Check sheet for the modelled part. Datum: model origin and axes. Units: mm. Coordinates: 2 decimals unless noted, no trailing zeros. Loops run counter-clockwise (first coordinate to the right, second up) from the corner with the lowest first, then second, coordinate; pieces in that order, holes last. Notation, with made-up numbers: (14.25, 22) - (36.25, 22) arc R27 ccw to (36.25, 49) - close; hole circle Ø11 at (0.5, 85). An arc over 180 degrees is marked (long way). Use a Markdown table: item, result. Add a question column.
1) Thickness scan on line 1 (X direction, y = 21, z = 1.3); line 2 (Y direction, x = -66, z = 1); line 3 (X direction, y = 5, z = 1.5). Record the ranges inside material, lowest first.
2) Draft check along X on faces 1 (the flat face through (-22, 14, 2)), 2 (the cylindrical face through (-20.43, 6.78, 0.99)), 3 (the flat face through (27.186, 14, 1)), 4 (the flat face through (-70.814, 14, 1)). Enter one of: pulls with the +X half, pulls with the -X half, needs draft (parallel to the pull), parting line crosses it, or undercut.
3) Sectioned sample at A-A, the plane x = -22. Enter the section's corners in (y, z).
4) Go/stop test with a flat-tipped pin: P1, Ø2.5, axis at x = -21.81, y = 6.2, coming from the +Z side. Record where the tip stops, or that it passes through.
Autodesk Inventor part; units mm, degrees
ref_plane "YZ Plane" through (0, 0, 0) normal (1, 0, 0) x (0, 1, 0)
ref_plane "XZ Plane" through (0, 0, 0) normal (0, 1, 0) x (-1, 0, 0)
ref_plane "XY Plane" through (0, 0, 0) normal (0, 0, 1) x (1, 0, 0)
sketch "Sketch1" plane through (0, 0, 0) normal (0, 0, 1) x (1, 0, 0)
  line L0 (27.1862, 25.2035) -> (-70.8138, 25.2035)
  line L1 (-70.8138, 25.2035) -> (-70.8138, 2.2035)
  line L2 (-70.8138, 2.2035) -> (27.1862, 2.2035)
  line L3 (27.1862, 2.2035) -> (27.1862, 25.2035)
  line L4 (27.1862, 25.2035) -> (27.1862, 21.2035)
  line L5 (27.1862, 21.2035) -> (23.1862, 21.2035)
  circle A0 centre (23.1862, 21.2035) radius 1.5
  line L6 (-70.8138, 25.2035) -> (-70.8138, 21.2035)
  line L7 (-70.8138, 21.2035) -> (-66.8138, 21.2035)
  circle A1 centre (-66.8138, 21.2035) radius 1.5
  line L8 (-21.8138, 2.2035) -> (-21.8138, 6.2035)
  circle A2 centre (-21.8138, 6.2035) radius 1.5
  point P0 (0, 0)
  dimension "d0" = 98
  dimension "d1" = 23
  dimension "d2" = 4
  dimension "d3" = 4
  dimension "d4" = 3
  dimension "d5" = 4
  dimension "d6" = 4
  dimension "d7" = 3
  dimension "d8" = 4
  dimension "d9" = 3
extrude "Extrusion1" add sketch "Sketch1" along normal blind 2
properties part number "konektor kort"
Solved:
| question | item | result |
|---|---|---|
| 1 | line 1 | x = -70.81 to -68.3, -65.33 to 21.7, 24.67 to 27.19 |
| 1 | line 2 | y = 2.2 to 19.94, 22.46 to 25.2 |
| 1 | line 3 | x = -70.81 to -22.71, -20.92 to 27.19 |
| 2 | face 1 | needs draft |
| 2 | face 2 | undercut |
| 2 | face 3 | pulls with the +X half |
| 2 | face 4 | pulls with the -X half |
| 3 | outline | (2.2, 0) - (4.72, 0) - (4.72, 2) - (2.2, 2) - close; (7.69, 0) - (25.2, 0) - (25.2, 2) - (7.69, 2) - close |
| 4 | P1 | passes through |
